Build history of the part. All positions in model axes, mm. A direction names the side the tool comes from. Round coordinates to 2 decimals unless told otherwise and drop trailing zeros. Write each loop counter-clockwise with the first axis right and the second up, starting at its lowest first coordinate (ties: lowest second). Pieces come first, ordered by that corner, then holes. Notation, with made-up numbers: M -21,22.5 L 26,22.5 A25 ccw 26,60.5 Z; hole C 10,85.5 d9. An arc over 180 degrees is marked long. Use a Markdown table: item, result.
Autodesk Inventor part; units mm, degrees
ref_plane "XZ Plane" through (0, 0, 0) normal (0, 1, 0) x (-1, 0, 0)
sketch "スケッチ1" plane through (0, 0, 0) normal (0, 0, 1) x (1, 0, 0)
  arc A0 (0, 35) -> (0, -35) centre (0, 0) ccw
  line L0 (0, 35) -> (0, -35)
  dimension "d0" = 70
revolve "回転1" add sketch "スケッチ1" angle 360 about axis through (0, 35, 0) along (0, -1, 0)
sketch "スケッチ2" plane through (0, 0, 0) normal (0, 0, 1) x (1, 0, 0)
  circle A0 centre (0, 0) radius 25
  dimension "d2" = 50
extrude "押し出し1" add sketch "スケッチ2" along normal blind 50
sketch "スケッチ3" plane through (0, 0, 0) normal (1, 0, 0) x (0, 1, 0)
  circle A0 centre (0, 0) radius 15
  dimension "d5" = 30
extrude "押し出し2" add sketch "スケッチ3" along normal mid plane 100
properties part number "UpperlegY"
Q1. Which spindle directions (+Z, -Z, +X, -X, +Y, -Y) get a long thin tool onto all of the face, cutting with end or side? Do faces 1 (the cylindrical face through (-40.683, -14.985, 0.66)), 2 (the cylindrical face through (40.683, 13.856, 5.745)), 3 (the cylindrical face through (23.846, -7.509, 37.069)). Say none if no direction does.
Response values:
| item | result |
|---|---|
| face 1 | -X |
| face 2 | +X |
| face 3 | +Z |
Q2. Cut at A-A on z = 0. Give the cut face in (x, y).
Response values:
| item | result |
|---|---|
| outline | M -50,-15 L -31.62,-15 A35 ccw 31.62,-15 L 50,-15 L 50,15 L 31.62,15 A35 ccw -31.62,15 L -50,15 Z |
Q3. Drop flat-ended pins along their axis: P1, Ø1.5, axis at x = -16, y = 19, coming from the -Z side; P2, Ø5, axis at x = -3, z = -19, coming from the -Y side; P3, Ø8, axis at x = 24.5, y = -18, coming from the +Z side. Give the stop position or say it passes through.
Response values:
| item | result |
|---|---|
| P1 | stops at z = -25.39 |
| P2 | stops at y = -30.74 |
| P3 | stops at z = 22.98 |
Q4. Cut at C-C on x = 0. Give the cut face in (y, z), and give its area (3 significant figures).
Response values:
| item | result |
|---|---|
| outline | M -25,24.49 A35 ccw long 25,24.49 L 25,50 L -25,50 Z |
| area | 4,760 mm2 |
Q5. Cut at D-D on x = -39. Give the cut face in (y, z).
Response values:
| item | result |
|---|---|
| outline | C 0,0 d30 |
Q6. Drill centre lines: L1, parallel to X at y = 10.5, z = 45; L2, parallel to X at y = -20.5, z = -13; L3, parallel to Y at x = 5, z = 37. Where is each one in solid material? Low to high.
Response values:
| item | result |
|---|---|
| L1 | x = -22.69 to 22.69 |
| L2 | x = -25.21 to 25.21 |
| L3 | y = -24.49 to 24.49 |
Q7. Cut at B-B on y = 0. Give the cut face in (x, z), and give its area (3 significant figures).
Response values:
| item | result |
|---|---|
| outline | M -50,-15 L -31.62,-15 A35 ccw 31.62,-15 L 50,-15 L 50,15 L 31.62,15 A35 ccw 25,24.49 L 25,50 L -25,50 L -25,24.49 A35 ccw -31.62,15 L -50,15 Z |
| area | 5,730 mm2 |
